The figure shows three views and two pictorial views of one solid part (mm, origin at its lowest corner). Answer the questions. A direction names the side the tool comes from. Give positions to 0.01 mm unless a question says otherwise; leave off trailing zeros. Order: outer loops, then holes, each group sorted by start corner. A loop starts at its lowest first (then second) coordinate and runs counter-clockwise, first axis right, second up. Notation, with made-up numbers: (44.5, 39.25) - (75.5, 39.25) arc R6 cw to (75.5, 49.25) - close; hole circle Ø1 at (20, 35.5). An arc over 180 degrees is marked (long way). Return JSON: item names as keys, results as strings. Group by question number.
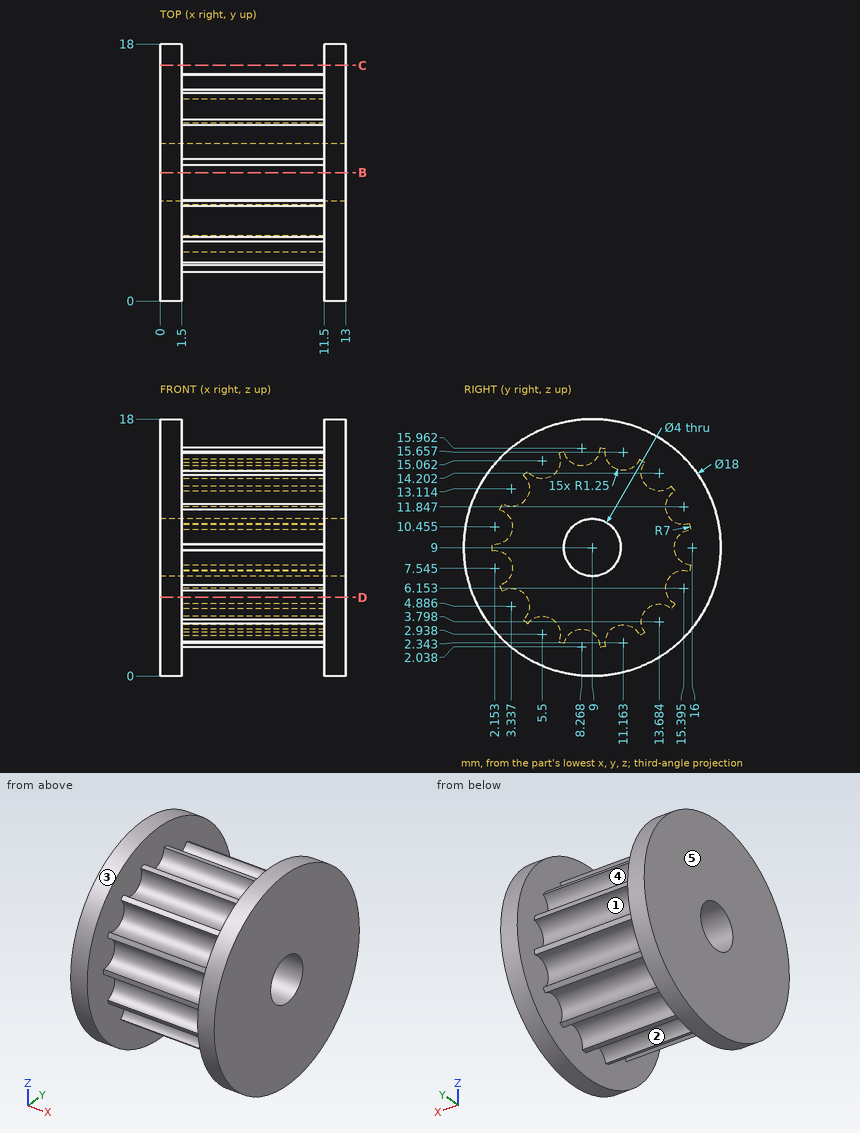
1. The part is cut by section D-D (z = 5.5). Give the vertices of the cut face in (x, y) (1 decimal), and give its area (3 significant figures).
2. The part is cut by section B-B (y = 9). Give the vertices of the cut face in (x, z).
3. Each of these flat-tipped pins is pushed along its axis until it touches: pin 1 (1.5 mm diameter, centred on x = 2.5, y = 9, fed in from +Z); pin 2 (1 mm diameter, centred on x = 6.5, y = 2.5, fed in from +Z); pin 3 (5 mm diameter, centred on x = 7.5, z = 10.5, fed in from +Y). Where does it stop, or does it pass through?
4. Determine the mould class of the marked faces 1, 2 and 3 for opening direction Y: released by +Y, released by -Y, zero draft, split by the parting line, or undercut.
5. Consider probe 1 along Z at (x, y) = (8.75, 9); probe 2 along X at (y, z) = (13.25, 1.25); probe 3 along Y at (x, z) = (9.5, 9). Determine where each line is inside the solid, lowest interval first. Write a range as from..to.
6. The part is cut by section C-C (y = 16.5). Give the vertices of the cut face in (x, z) (1 decimal).
7. A tool of negligible diameter and unlimited length cuts with its end or side. For the marked faces 4 and 5, from which of +Z, -Z, +X, -X, +Y, -Y can it reach the whole face along a straight path? Write none if from no direction.
Answers:
{
 "1": {"outline": "(0, 0.7) - (1.5, 0.7) - (1.5, 4.4) - (11.5, 4.4) - (11.5, 0.7) - (13, 0.7) - (13, 17.3) - (11.5, 17.3) - (11.5, 14.3) - (1.5, 14.3) - (1.5, 17.3) - (0, 17.3) - close", "area": "149 mm^2"},
 "2": {"outline": "(0, 0) - (1.5, 0) - (1.5, 3.05) - (11.5, 3.05) - (11.5, 0) - (13, 0) - (13, 7) - (0, 7) - close; (0, 11) - (13, 11) - (13, 18) - (11.5, 18) - (11.5, 14.95) - (1.5, 14.95) - (1.5, 18) - (0, 18) - close"},
 "3": {"pin 1": "stops at z = 15.98", "pin 2": "stops at z = 12.04", "pin 3": "stops at y = 15.89"},
 "4": {"face 1": "released by +Y", "face 2": "undercut", "face 3": "split by the parting line"},
 "5": {"probe 1": "z = 3.05..7, 11..14.95", "probe 2": "x = 0..1.5, 11.5..13", "probe 3": "y = 2..7, 11..14.75"},
 "6": {"outline": "(0, 4) - (1.5, 4) - (1.5, 14) - (0, 14) - close; (11.5, 4) - (13, 4) - (13, 14) - (11.5, 14) - close"},
 "7": {"face 4": "none", "face 5": "+Z, -Z, -X, +Y, -Y"}
}
